```python
from build123d import *

# Parameters (mm, degrees)
SKETCH1_W           = 30
SKETCH1_H           = 15
BOSS_EXTRUDE1_DEPTH = 3
CUT_EXTRUDE1_START  = -4
SKETCH2_R           = 3.9
CUT_EXTRUDE1_DEPTH  = 5


with BuildPart() as part:
    # Sketch1 → Boss-Extrude1 (new body)
    with BuildSketch(Plane(origin=(0, 0, 0), x_dir=(1, 0, 0), z_dir=(0, 1, 0))):
        Rectangle(SKETCH1_W, SKETCH1_H)
    extrude(amount=BOSS_EXTRUDE1_DEPTH)

    # Sketch2 → Cut-Extrude1 (cut)
    with BuildSketch(Plane(origin=(0, 3, 0), x_dir=(1, 0, 0), z_dir=(0, 1, 0)).offset(CUT_EXTRUDE1_START)):
        with Locations((-6.5, 0)):
            Circle(SKETCH2_R)
    cut_extrude1 = extrude(amount=CUT_EXTRUDE1_DEPTH, mode=Mode.SUBTRACT)

    # Mirror1: Cut-Extrude1 across plane
    add(cut_extrude1.mirror(Plane(origin=(0, 0, 0), x_dir=(0, 0, 1), z_dir=(1, 0, 0))), mode=Mode.SUBTRACT)


solid = part.part
```
Design review of the part built by this model. Coordinates are the model's own, in mm. Coordinates: 2 decimals unless noted, no trailing zeros. Loops run counter-clockwise (first coordinate to the right, second up) from the corner with the lowest first, then second, coordinate; pieces in that order, holes last.
Q1. The part is to be moulded in two halves that separate along X. For faces 1 (the face through (0, 0, 0)), 2 (the face through (15, 1, 0)), 3 (the face through (-2.78, 1.48, -1.17)), say which applies: +X half, -X half, draft (parallel to the pull), parting line (faces both ways), or undercut.
Reported:
face 1: draft
face 2: +X half
face 3: undercut
Q2. For pin 1 (9 mm diameter, centred on x = 6.5, z = 0, fed in from -Y), flat-tipped, find the tip position at first contact; note if it passes through.
Reported:
pin 1: stops at y = 0
Q3. To check wall thickness, follow line 1 (Z direction, x = 6.5, y = 2.25); line 2 (X direction, y = 1.4, z = -2.5); line 3 (Z direction, x = -5, y = 2.15). State the ranges of each line that lie inside material, in increasing order.
Reported:
line 1: z = -7.5 to -3.9, 3.9 to 7.5
line 2: x = -15 to -9.49, -3.51 to 3.51, 9.49 to 15
line 3: z = -7.5 to -3.6, 3.6 to 7.5
Q4. We need section B-B on x = 6.5. State the section outline as (y, z) points.
Reported:
outline: (0, -7.5) - (3, -7.5) - (3, -3.9) - (0, -3.9) - close; (0, 3.9) - (3, 3.9) - (3, 7.5) - (0, 7.5) - close
Q5. We need section C-C on y = 0.95. State the section outline as (x, z) points, and give its area (3 significant figures).
Reported:
outline: (-15, -7.5) - (15, -7.5) - (15, 7.5) - (-15, 7.5) - close; hole circle Ø7.8 at (-6.5, 0); hole circle Ø7.8 at (6.5, 0)
area: 354 mm2
Q6. We need section A-A on z = 0. State the section outline as (x, y) points, and give its area (3 significant figures).
Reported:
outline: (-15, 0) - (-10.4, 0) - (-10.4, 3) - (-15, 3) - close; (-2.6, 0) - (2.6, 0) - (2.6, 3) - (-2.6, 3) - close; (10.4, 0) - (15, 0) - (15, 3) - (10.4, 3) - close
area: 43.2 mm2
